```python
from build123d import *

# Parameters (mm, degrees)
F0_W     = 60
F0_H     = 110
F1_DEPTH = 80
F2_W     = 35
F2_H     = 50
F3_DEPTH = 110
F4_W     = 25
F4_H     = 40
F5_DEPTH = 30
F6_R     = 5
F7_DEPTH = 25


with BuildPart() as f1:
    # F0 (on Top) → F1 (new body)
    with BuildSketch(Plane.XY):
        with Locations((-28.960537, 38.087605)):
            Rectangle(F0_W, F0_H)
    extrude(amount=F1_DEPTH)

    # F2 (on face) → F3 (cut)
    with BuildSketch(Plane.XZ.offset(16.912395)):
        with Locations((-16.460537, 55)):
            Rectangle(F2_W, F2_H)
    extrude(amount=-F3_DEPTH, mode=Mode.SUBTRACT)

    # F4 (on face) → F5 (cut)
    with BuildSketch(Plane.XY.offset(30)):
        with Locations((-11.460537, 38.087605)):
            Rectangle(F4_W, F4_H)
    extrude(amount=-F5_DEPTH, mode=Mode.SUBTRACT)

    # F6 (on face) → F7 (cut)
    with BuildSketch(Plane.YZ.offset(-33.960537)):
        with Locations((13.087605, 55)):
            Circle(F6_R)
        with Locations((63.087605, 55)):
            Circle(F6_R)
    extrude(amount=-F7_DEPTH, mode=Mode.SUBTRACT)


solid = f1.part
```
Build history of the part. All positions in model axes, mm. A direction names the side the tool comes from. Coordinates: 2 decimals unless noted, no trailing zeros. Order: outer loops, then holes, each group sorted by start corner. A loop starts at its lowest first (then second) coordinate and runs counter-clockwise, first axis right, second up. Notation, with made-up numbers: (-32.75, -15) -> (-3.75, -15) arc R21 ccw to (-3.75, -1) -> close; hole circle Ø8 at (-12, -14). An arc over 180 degrees is marked (long way). Answer in a Markdown table with one row per item. Add a question column.
Q1. Band-saw the part on D-D, the plane y = 45.5. List the corners of the cut face in (x, z).
Q2. Which spindle directions (+Z, -Z, +X, -X, +Y, -Y) get a long thin tool onto all of the face, cutting with end or side? Do faces 4 (the face through (-46.286, 12.437, 59.957)), 5 (the face through (-24.5, 37.3, 30)), 6 (the face through (-12, 18.088, 15)). Say none if no direction does.
Q3. Band-saw the part on C-C, the plane z = 11. List the corners of the cut face in (x, y), then the cut area to 3 significant figures.
Q4. Wall check: line 1 along Y through (x, z) = (-14, 12); line 2 along Z through (x, y) = (-30.5, 1); line 3 along X through (y, z) = (43.5, 45). Give the ranges that are in metal, low to high. Write a range as [from, to].
Q5. Drop flat-ended pins along their axis: pin 1 (8 mm diameter, centred on y = 63.09, z = 55, fed in from +X); pin 2 (12 mm diameter, centred on x = -28, y = 11, fed in from +Z); pin 3 (10 mm diameter, centred on y = 29, z = 54, fed in from +X); pin 4 (2 mm diameter, centred on x = -28, y = 77, fed in from +Z). Give the stop position or say it passes through.
Q6. Mould opens along Y. For faces 1 (the face through (-29, 39, 0)), 2 (the face through (-36, -16.912, 31)), 3 (the face through (-12, 58.088, 15)) say: +Y half, -Y half, draft (parallel to the pull), parting line (faces both ways), or undercut.
Q7. Band-saw the part on B-B, the plane y = 62. List the corners of the cut face in (x, z), then the cut area to 3 significant figures.
Q8. Band-saw the part on A-A, the plane z = 55. List the corners of the cut face in (x, y).
Answers follow:
| question | item | result |
|---|---|---|
| 1 | outline | (-58.96, 0) -> (-23.96, 0) -> (-23.96, 30) -> (-33.96, 30) -> (-33.96, 80) -> (-58.96, 80) -> close |
| 2 | face 4 | +X, -X |
| 2 | face 5 | +Z, +X, +Y, -Y |
| 2 | face 6 | +Z, -Z, +X |
| 3 | outline | (-58.96, -16.91) -> (1.04, -16.91) -> (1.04, 18.09) -> (-23.96, 18.09) -> (-23.96, 58.09) -> (1.04, 58.09) -> (1.04, 93.09) -> (-58.96, 93.09) -> close |
| 3 | area | 5,600 mm^2 |
| 4 | line 1 | [-16.91, 18.09], [58.09, 93.09] |
| 4 | line 2 | [0, 30] |
| 4 | line 3 | [-58.96, -33.96] |
| 5 | pin 1 | through |
| 5 | pin 2 | z = 80 |
| 5 | pin 3 | x = -33.96 |
| 5 | pin 4 | z = 30 |
| 6 | face 1 | draft |
| 6 | face 2 | -Y half |
| 6 | face 3 | undercut |
| 7 | outline | (-58.96, 0) -> (1.04, 0) -> (1.04, 30) -> (-33.96, 30) -> (-33.96, 50.12) -> (-58.96, 50.12) -> close; (-58.96, 59.88) -> (-33.96, 59.88) -> (-33.96, 80) -> (-58.96, 80) -> close |
| 7 | area | 2,810 mm^2 |
| 8 | outline | (-58.96, -16.91) -> (-33.96, -16.91) -> (-33.96, 8.09) -> (-58.96, 8.09) -> close; (-58.96, 18.09) -> (-33.96, 18.09) -> (-33.96, 58.09) -> (-58.96, 58.09) -> close; (-58.96, 68.09) -> (-33.96, 68.09) -> (-33.96, 93.09) -> (-58.96, 93.09) -> close |
